Could you check a few things on this model? Use its own coordinates, in mm. A direction names the side the tool comes from. Give positions to 0.01 mm unless a question says otherwise; leave off trailing zeros. Loops run counter-clockwise (first coordinate to the right, second up) from the corner with the lowest first, then second, coordinate; pieces in that order, holes last. Notation, with made-up numbers: M -26,61 L 12,61 A21 ccw 12,97 Z; hole C 38.25,15 d5. An arc over 180 degrees is marked long. Answer in a Markdown table with one row per item. Add a question column.
1. I'm going to push flat-ended pins straight in: pin 1 Ø1.5 at (x, y) = (14, 2) entering from +Z; pin 2 Ø4 at (y, z) = (1, 0.5) entering from -X; pin 3 Ø5 at (x, z) = (5.5, -2) entering from +Y (3 decimals). Where does each tip first touch, or does it pass through?
2. Thinking about a two-plate mould opening in Y: for faces 5 (the flat face through (-1.27, -4, -3)), 6 (the flat face through (-3.649, -4.144, -2.348)), 7 (the flat face through (-5.613, 0, 0)), 8 (the flat face through (-3.649, 4.144, 2.348)), which applies, released by +Y, released by -Y, zero draft, split by the parting line, or undercut?
3. I need wall thicknesses on line 1 along Z through (x, y) = (-5.75, 0); line 2 along X through (y, z) = (4.5, 2.75); line 3 along X through (y, z) = (2.75, -2). Which ranges of each line are inside material? Lowest first, please. Write a range as from..to.
4. Which directions (+Z, -Z, +X, -X, +Y, -Y) give clear straight access to the entire face, cutting with the end or side of a thin tool? Please do faces 1 (the cylindrical face through (10.33, -0.69, 3.1)), 2 (the flat face through (-3.65, -4.11, 2.41)), 3 (the flat face through (-4, 0, -4.762)), 4 (the flat face through (-4, 0, 4.762)).
5. If we section it at C-C on x = -4: List the corners of the cut face in (y, z) for me.
6. If we section it at A-A on x = 19.5: List the corners of the cut face in (y, z) for me (3 decimals), then the cut area to 3 significant figures.
7. If we section it at B-B on z = 5.5: List the corners of the cut face in (x, y) for me.
Autodesk Inventor part; units mm, degrees
ref_plane "IDS_WORKPLANE{1}" through (-6.096, 0, 0) normal (-1, 0, 0) x (0, 0, -1)
ref_plane "Work Plane3" through (7, 0, 0) normal (0, 0, -1) x (1, 0, 0)
ref_plane "YZ Plane" through (0, 0, 0) normal (1, 0, 0) x (0, 1, 0)
sketch "Sketch1" plane through (0, 0, 0) normal (0, 0, 1) x (1, 0, 0)
  line L0 (-1.27, 6.604) -> (-1.27, 0)
  line L1 (-1.27, 0) -> (25.4, 0)
  line L2 (25.4, 0) -> (25.4, 3.175)
  line L3 (25.4, 3.175) -> (0, 3.175)
  line L4 (0, 3.175) -> (0, 6.604)
  line L5 (-6.604, 0) -> (30.734, 0)
  line L6 (0, -1.3208) -> (0, 7.9248)
  line L7 (0, 6.604) -> (-1.27, 6.604)
  dimension "d1" = 1.27
  dimension "d2" = 6.35
  dimension "d3" = 25.4
  dimension "d22" = 13.208
revolve "Body" add sketch "Sketch1" angle 360 about axis through (-1.27, 0, 0) along (1, 0, 0)
sketch "Sketch2" plane through (-1.27, 0, 0) normal (-1, 0, 0) x (0, 0, 1)
  line L0 (0, 5.4993) -> (4.7625, 2.7496)
  line L1 (4.7625, 2.7496) -> (4.7625, -2.7496)
  line L2 (4.7625, -2.7496) -> (0, -5.4993)
  line L3 (0, -5.4993) -> (-4.7625, -2.7496)
  line L4 (-4.7625, -2.7496) -> (-4.7625, 2.7496)
  line L5 (-4.7625, 2.7496) -> (0, 5.4993)
  circle A0 centre (0, 0) radius 6.604
  dimension "d11" = 9.525
extrude "Head" add sketch "Sketch2" along normal blind 4.826 contours L0 L1 L2 L3 L4 L5
ref_plane "IDS_WORKPLANE{1}" through (-6.096, 0, 0) normal (-1, 0, 0) x (0, 0, -1)
sketch "Sketch3" plane through (-6.096, 0, 0) normal (-1, 0, 0) x (0, 0, -1)
  circle A0 centre (0, 0) radius 3.81
  point P0 (0, 0)
  dimension "d15" = 7.62
extrude "Indent" cut sketch "Sketch3" against normal blind 0.4826
thread "Thread"
sketch "Sketch4" plane through (0, 0, 0) normal (0, 0, 1) x (1, 0, 0)
  line L0 (-6.096, 4.7625) -> (-6.096, 5.4993)
  line L1 (-6.096, 5.4993) -> (-5.5092, 5.4993)
  line L2 (-6.096, 5.4993) -> (-6.096, 2.7496)
  line L3 (-7.4557, 0) -> (1.9883, 0)
  line L4 (-1.27, 5.4993) -> (-6.096, 5.4993)
  arc A0 (-5.5092, 5.4993) -> (-6.096, 4.7625) centre (0.6392, 0) ccw
  dimension "d21" = 9.525
  dimension "d23" = 8.2489
revolve "Chamfer1" cut sketch "Sketch4" angle 360 about axis through (-10, 0, 0) along (1, 0, 0)
chamfer "Chamfer2" distance 0.635 distance2 4.445 1 edges at (25.4, -3.175, 0) measured on face at (25.4, -0.5202, -0.7796)
ref_plane "Work Plane3" through (7, 0, 0) normal (0, 0, -1) x (1, 0, 0)
equation "\"d1\" = SD"
equation "\"d2\" = NND"
equation "\"d3\" = NLG"
equation "\"d22\" = SD2"
equation "\"d11\" = SW"
equation "\"d12\" = KOH"
equation "\"d15\" = SD3"
equation "\"d16\" = SB"
equation "\"d21\" = SW"
equation "\"d23\" = 0.866025 * SW"
equation "\"d6\" = GEL"
equation "\"d19\" = -0.5 * GD2 + 0.5 * NND"
equation "\"d20\" = SPTZ"
equation "\"NLG\" = 25.4"
equation "\"NND\" = 6.35"
equation "\"KOH\" = 4.826"
equation "\"GEL\" = 25.4"
equation "\"SW\" = 9.525"
equation "\"GD2\" = 5.08"
equation "\"SPTZ\" = 4.445"
equation "\"SD3\" = 0.8 * SW"
equation "\"SB\" = 0.1 * KOH"
equation "\"SD2\" = 13.208"
equation "\"SD\" = 1.27"
equation "\"GD1\" = 5.08"
equation "\"THREADDIA\" = 6.35"
equation "\"TOA\" = 30deg"
equation "\"E0\" = 10.99852"
properties part number "am-1182" material "Steel, Mild"
Results:
| question | item | result |
|---|---|---|
| 1 | pin 1 | z = 2.92 |
| 1 | pin 2 | x = -5.61 |
| 1 | pin 3 | y = 3.175 |
| 2 | face 5 | zero draft |
| 2 | face 6 | released by -Y |
| 2 | face 7 | undercut |
| 2 | face 8 | released by +Y |
| 3 | line 1 | -4.76..-3.81, 3.81..4.76 |
| 3 | line 2 | -1.27..0 |
| 3 | line 3 | -5.61..0 |
| 4 | face 1 | +X |
| 4 | face 2 | +Z, -X, -Y |
| 4 | face 3 | -Z, -X, +Y, -Y |
| 4 | face 4 | +Z, -X, +Y, -Y |
| 5 | outline | M -5.5,0 L -2.75,-4.76 L 2.75,-4.76 L 5.5,0 L 2.75,4.76 L -2.75,4.76 Z |
| 6 | outline | C 0,0 d6.35 |
| 6 | area | 31.7 mm2 |
| 7 | outline | M -1.27,-3.66 L 0,-3.66 L 0,3.66 L -1.27,3.66 Z |
